```python
from build123d import *

# Parameters (mm, degrees)
SKETCH1_R           = 38.25
BOSS_EXTRUDE1_DEPTH = 250
CUT_EXTRUDE2_DEPTH  = 50
SKETCH4_R           = 35
SKETCH4_R_2         = 15
BOSS_EXTRUDE2_DEPTH = 50
BOSS_EXTRUDE3_START = 75
SKETCH5_R           = 15
BOSS_EXTRUDE3_DEPTH = 75


with BuildPart() as part:
    # Sketch1 → Boss-Extrude1 (new body)
    with BuildSketch(Plane.XY):
        Circle(SKETCH1_R)
    boss_extrude1 = extrude(amount=BOSS_EXTRUDE1_DEPTH)

    # Sketch3 → Cut-Extrude2 (cut)
    with BuildSketch(Plane.XY.offset(250)):
        with BuildLine():
            Line((-8.5, 26.940907557), (-8.5, 33.25))
            Line((-8.5, 33.25), (8.5, 33.25))
            Line((8.5, 33.25), (8.5, 26.940907557))
            ThreePointArc((8.5, 26.940907557), (0, -28.25), (-8.5, 26.940907557))
        make_face()
    cut_extrude2 = extrude(amount=-CUT_EXTRUDE2_DEPTH, mode=Mode.SUBTRACT)

    # Mirror1: Boss-Extrude1, Cut-Extrude2 across plane
    add(boss_extrude1.mirror(Plane.XY))
    add(cut_extrude2.mirror(Plane.XY), mode=Mode.SUBTRACT)

    # Sketch4 → Boss-Extrude2 (add)
    with BuildSketch(Plane(origin=(0, 0, -250), x_dir=(-1, 0, 0), z_dir=(0, 0, -1))):
        Circle(SKETCH4_R)
        Circle(SKETCH4_R_2, mode=Mode.SUBTRACT)
    extrude(amount=-BOSS_EXTRUDE2_DEPTH)

    # Sketch5 → Boss-Extrude3 (add)
    with BuildSketch(Plane(origin=(0, 0, -200), x_dir=(-1, 0, 0), z_dir=(0, 0, -1)).offset(BOSS_EXTRUDE3_START)):
        Circle(SKETCH5_R)
    extrude(amount=-BOSS_EXTRUDE3_DEPTH)


solid = part.part
```
Model file for the job. Use its own axes, mm. A direction names the side the tool comes from. Give positions to 0.01 mm unless a question says otherwise; leave off trailing zeros. Order: outer loops, then holes, each group sorted by start corner. A loop starts at its lowest first (then second) coordinate and runs counter-clockwise, first axis right, second up.
1) Saw through at D-D, the plane x = -20. Write the cut outline in (y, z), then the cut area to 3 significant figures.
2) Saw through at B-B, the plane x = 0. Write the cut outline in (y, z), then the cut area to 3 significant figures.
3) Wall check: probe 1 along Y at (x, z) = (0, 221); probe 2 along Z at (x, y) = (-29, -12.5); probe 3 along Z at (x, y) = (3, -5.5). Give the ranges that are in metal, low to high.
4) Mould opens along X. For faces 3 (the flat face through (-1, -16, -250)), 4 (the flat face through (0, 33.25, 225)), 5 (the cylindrical face through (14.985, 0.66, -262.675)) say: +X half, -X half, draft (parallel to the pull), parting line (faces both ways), or undercut.
5) Saw through at A-A, the plane y = 0. Write the cut outline in (x, z).
6) Saw through at C-C, the plane z = -212. Write the cut outline in (x, y).
7) Pin check, flat tips, straight feed: pin 1 (1 mm diameter, centred on x = -15.5, y = 5.5, fed in from -Z); pin 2 (18.5 mm diameter, centred on x = 2.5, z = 226, fed in from -Y); pin 3 (1.9 mm diameter, centred on y = 29.5, z = 214, fed in from +X); pin 4 (10 mm diameter, centred on y = 2, z = -158, fed in from -X). Stop position of each tip, or through.
8) 3-axis set-ups, long thin cutter, end or side, ignore diameter. For faces 1 (the cylindrical face through (1.121, -28.228, 225.35)), 2 (the flat face through (-23, -17, 250)): which of +Z, -Z, +X, -X, +Y, -Y reach the whole face in a straight line?
Computed:
1. outline: (-32.6, -250) - (32.6, -250) - (32.6, 250) - (19.95, 250) - (19.95, 200) - (-19.95, 200) - (-19.95, 250) - (-32.6, 250) - close
1. area: 30,600 mm2
2. outline: (-38.25, -250) - (-15, -250) - (-15, -275) - (15, -275) - (15, -250) - (38.25, -250) - (38.25, 250) - (33.25, 250) - (33.25, 200) - (-28.25, 200) - (-28.25, 250) - (-38.25, 250) - close
2. area: 35,900 mm2
3. probe 1: y = -38.25 to -28.25, 33.25 to 38.25
3. probe 2: z = -250 to 250
3. probe 3: z = -275 to 200
4. face 3: draft
4. face 4: undercut
4. face 5: parting line
5. outline: (-38.25, -250) - (-15, -250) - (-15, -275) - (15, -275) - (15, -250) - (38.25, -250) - (38.25, 250) - (28.25, 250) - (28.25, 200) - (-28.25, 200) - (-28.25, 250) - (-38.25, 250) - close
6. outline: circle Ø76.5 at (0, 0)
7. pin 1: stops at z = -250
7. pin 2: stops at y = -38.25
7. pin 3: stops at x = 25.46
7. pin 4: stops at x = -38.25
8. face 1: +Z
8. face 2: +Z, +X, -X, +Y, -Y
